Here's how the part is built. I have some questions about the finished solid (model axes, mm). A direction names the side the tool comes from. Give positions to 0.01 mm unless a question says otherwise; leave off trailing zeros. Write each loop counter-clockwise with the first axis right and the second up, starting at its lowest first coordinate (ties: lowest second). Pieces come first, ordered by that corner, then holes. Notation, with made-up numbers: (2.25, -35.75) - (47.25, -35.75) arc R13 ccw to (47.25, -24.75) - close; hole circle Ø1 at (41.25, 79). An arc over 180 degrees is marked (long way). Use a Markdown table: item, result.
Autodesk Inventor part; units mm, degrees
ref_plane "YZ Plane" through (0, 0, 0) normal (1, 0, 0) x (0, 1, 0)
ref_plane "XZ Plane" through (0, 0, 0) normal (0, 1, 0) x (-1, 0, 0)
ref_plane "XY Plane" through (0, 0, 0) normal (0, 0, 1) x (1, 0, 0)
sketch "Sketch1" plane through (0, 0, 0) normal (0, 1, 0) x (-1, 0, 0)
  circle A0 centre (0, 0) radius 23
  circle A1 centre (0, 0) radius 20
  dimension "d0" = 3
  dimension "d1" = 40
extrude "Extrusion1" add sketch "Sketch1" along normal blind 2680.4
sketch "Sketch2" plane through (0, 0, 0) normal (0, 0, 1) x (1, 0, 0)
  line L0 (23, 2680.4) -> (-23, 2680.4)
  point P0 (0, 0)
  point P1 (0, 2673.4)
  point P2 (0, 2680.4)
  dimension "d4" = 7
hole "Hole1" [suppressed]
sketch3d "3D Sketch1"
sketch "Sketch3" plane through (0, 0, 0) normal (0, -1, 0) x (1, 0, 0)
  circle A0 centre (0, 0) radius 20
  circle A1 centre (0, 0) radius 23
sweep "Sweep1" [suppressed]
sketch "Sketch4" plane through (162.5, -96, -92.5) normal (0, 0, -1) x (-1, 0, 0)
  circle A0 centre (0, 0) radius 23
  point P0 (162.5, 96)
  point P1 (-22.6674, -3.8973)
extrude "Extrusion2" [suppressed]
sketch "Sketch5" plane through (0, 0, 0) normal (0, -1, 0) x (1, 0, 0)
  circle A0 centre (0, 0) radius 20
  circle A1 centre (0, 0) radius 23
sketch3d "3D Sketch2"
  spline S0 degree 3 poles (0, 0, 0) (0, -80, 0) (0, -80, 405) (0, -160, 405) knots 1 1 1 1 2 2 2 2
  dimension "d28" = 80
  dimension "d29" = 405
  dimension "d30" = 80
sweep "Sweep2" add profiles "Sketch5" path "3D Sketch2"
sketch "Sketch6" plane through (0, -160, 405) normal (0, -1, 0) x (1, 0, 0)
  spline S0 degree 6 poles (20, 0) (20, -33.2309) (-21.091, -38.0022) (-54.9823, 0) (-21.091, 38.0022) (20, 33.2309) (20, 0) knots 0 0 0 0 0 0 0 1 1 1 1 1 1 1 weights 1.669078 1.03673 1.038347 0.853534 1.038347 1.03673 1.669078
  circle A0 centre (0, 0) radius 23
  point P0 (0, -405)
  point P1 (23, 0)
extrude "Extrusion3" add sketch "Sketch6" along normal blind 40
properties part number "Top_End Pipe 1" material "PMMA Plastic"
Item 1: If we section it at A-A, the plane y = 2092.5: Write out the boundary of the cut face in (x, z).
Values:
| item | result |
|---|---|
| outline | circle Ø46 at (0, 0); hole circle Ø40 at (0, 0) |
Item 2: I need wall thicknesses on line 1 along Z through (x, y) = (1, 259); line 2 along X through (y, z) = (656.5, 0); line 3 along Z through (x, y) = (3, 1735). Which ranges of each line are inside material? Lowest first, please. Write a range as [from, to].
Values:
| item | result |
|---|---|
| line 1 | z = [-22.98, -19.97], [19.97, 22.98] |
| line 2 | x = [-23, -20], [20, 23] |
| line 3 | z = [-22.8, -19.77], [19.77, 22.8] |
Item 3: Thinking about a two-plate mould opening in Z: for faces 1 (the cylindrical face through (2.994, 1321.437, -22.804)), 2 (the flat face through (7, 2680.4, 19)), which applies, +Z half, -Z half, draft (parallel to the pull), parting line (faces both ways), or undercut?
Values:
| item | result |
|---|---|
| face 1 | parting line |
| face 2 | draft |
Item 4: For faces 3 (the cylindrical face through (12.365, -179.72, 385.606)), 4 (the flat face through (-5, -200, 385)), which set-ups out of +Z, -Z, +X, -X, +Y, -Y let a thin tool reach every point of the face, with its end or its side?
Values:
| item | result |
|---|---|
| face 3 | -Y |
| face 4 | +Z, -Z, +X, -X, -Y |
Item 5: Will these pins go through, and if not, where does the flat tip stop? pin 1 Ø1 at (x, y) = (-2, 1125) entering from -Z; pin 2 Ø6 at (x, y) = (-18, 1567) entering from +Z; pin 3 Ø10 at (x, y) = (1.5, 1672.5) entering from -Z.
Values:
| item | result |
|---|---|
| pin 1 | stops at z = -22.95 |
| pin 2 | stops at z = 17.44 |
| pin 3 | stops at z = -23 |
